For this review, take the finished solid that the model builds, in its own axes (mm). A direction names the side the tool comes from. Coordinates: 2 decimals unless noted, no trailing zeros. Order: outer loops, then holes, each group sorted by start corner. A loop starts at its lowest first (then second) coordinate and runs counter-clockwise, first axis right, second up.
from build123d import *

# Parameters (mm, degrees)
F1_DEPTH = 12.7
F2_R     = 12.7
F3_R     = 12.69999
F4_R     = 12.4821589041
F5_DEPTH = 31.75
F6_DEPTH = 12.7
F7_R     = 12.7
F8_R     = 12.69999


# Not quite as in the source:
# - a fillet or chamfer is up to 0.001 mm smaller than in the source, because OpenCascade refuses the exact size
# - the program builds the solid bodies; features that only make, move or delete a surface that nothing else refers to are left out


with BuildPart() as f1:
    # F0 (on Top) → F1 (new body)
    with BuildSketch(Plane.XY):
        Polygon((0, 25.4), (0, 0), (76.2, 0), (76.1904343963, 25.4), align=None)
    extrude(amount=F1_DEPTH)

    # F2
    f2_edges = [f1.edges().sort_by_distance(p)[0] for p in [
        (76.190434, 25.4, 6.35),
    ]]
    fillet(f2_edges, radius=F2_R)

    # F3 (radius 12.7 in the source; OpenCascade refuses exactly that, so slightly less here)
    f3_edges = [f1.edges().sort_by_distance(p)[0] for p in [
        (76.2, 0, 6.35),
    ]]
    fillet(f3_edges, radius=F3_R)

    # F4 (on Top) → F5 (join)
    with BuildSketch(Plane.XY):
        with Locations((14.5669719204, 12.8659298643)):
            Circle(F4_R)
    extrude(amount=-F5_DEPTH)

    # F6 (add): a face of the model
    f6_faces = [f1.faces().sort_by_distance(p)[0] for p in [
        (14.5669719204, 12.8659298643, -31.75),
    ]]
    extrude(f6_faces, amount=-F6_DEPTH)

    # F7
    f7_edges = [f1.edges().sort_by_distance(p)[0] for p in [
        (0, 0, 6.35),
    ]]
    fillet(f7_edges, radius=F7_R)

    # F8 (radius 12.7 in the source; OpenCascade refuses exactly that, so slightly less here)
    f8_edges = [f1.edges().sort_by_distance(p)[0] for p in [
        (0, 25.4, 6.35),
    ]]
    fillet(f8_edges, radius=F8_R)


solid = f1.part
1. Machinability: for faces 1 (the face through (72.572, 21.583, 6.439)), 2 (the face through (26.1, 8.09, -15.65)), which of the approach directions +Z, -Z, +X, -X, +Y, -Y give a long, thin tool a straight path to every point of the face, cutting with its end or side? Answer none if there is none.
Answer below:
face 1: +Z, -Z, +X, +Y
face 2: -Z
2. Take a section at D-D, the plane x = 36.5. Give the boundary of the cut face in (y, z), plus the area to 3 significant figures.
Answer below:
outline: (0, 0) - (25.4, 0) - (25.4, 12.7) - (0, 12.7) - close
area: 323 mm2
3. Clearance check with flat-ended pins moving along their axes: pin 1 Ø5 at (x, z) = (9, 6.5) entering from +Y; pin 2 Ø10 at (x, z) = (9, -9.5) entering from -Y; pin 3 Ø7.5 at (x, y) = (35.5, 18) entering from -Z. State where each tip first meets the part, or that it passes through.
Answer below:
pin 1: stops at y = 25.34
pin 2: stops at y = 0.4
pin 3: stops at z = 0
4. Take a section at B-B, the plane x = 25. Give the boundary of the cut face in (y, z).
Answer below:
outline: (0, 0) - (6.01, 0) - (6.01, -31.75) - (19.72, -31.75) - (19.72, 0) - (25.4, 0) - (25.4, 12.7) - (0, 12.7) - close
5. Take a section at C-C, the plane z = -26. Give the boundary of the cut face in (x, y), plus the area to 3 significant figures.
Answer below:
outline: circle Ø24.96 at (14.57, 12.87)
area: 489 mm2
6. Take a section at A-A, the plane y = 9.75. Give the boundary of the cut face in (x, z), plus the area to 3 significant figures.
Answer below:
outline: (0.35, 0) - (2.48, 0) - (2.48, -31.75) - (26.65, -31.75) - (26.65, 0) - (75.85, 0) - (75.85, 12.7) - (0.35, 12.7) - close
area: 1,730 mm2
7. To check wall thickness, follow L1, parallel to X at y = 13.25, z = -6; L2, parallel to Z at x = 41, y = 13.5; L3, parallel to Y at x = 20.5, z = -29.5. State the ranges of each line that lie inside material, in increasing order.
Answer below:
L1: x = 2.09 to 27.04
L2: z = 0 to 12.7
L3: y = 1.88 to 23.85
